from build123d import *

# Parameters (mm, degrees)
SKETCH1_R           = 1.755
SKETCH1_R_2         = 8
BOSS_EXTRUDE1_DEPTH = 3.175
SKETCH2_R           = 7.95936
SKETCH2_R_2         = 1.71436
BOSS_EXTRUDE2_DEPTH = 3.175


with BuildPart() as part:
    # Sketch1 → Boss-Extrude1 (new body)
    with BuildSketch(Plane.XY):
        Polygon((-50, 30), (-50, 33.175), (-70, 33.175), (-70, 30), (-90, 30), (-90, 33.175), (-110, 33.175), (-110, -33.175), (-90, -33.175), (-90, -30), (-70, -30), (-70, -33.175), (-50, -33.175), (-50, -30), (-30, -30), (-30, -33.175), (-10, -33.175), (-10, -30), (10, -30), (10, -33.175), (30, -33.175), (30, -30), (50, -30), (50, -33.175), (70, -33.175), (70, -30), (90, -30), (90, -33.175), (110, -33.175), (110, 33.175), (90, 33.175), (90, 30), (70, 30), (70, 33.175), (50, 33.175), (50, 30), (30, 30), (30, 33.175), (10, 33.175), (10, 30), (-10, 30), (-10, 33.175), (-30, 33.175), (-30, 30), align=None)
        with Locations((-65, -15)):
            Circle(SKETCH1_R, mode=Mode.SUBTRACT)
        with Locations((65, -15)):
            Circle(SKETCH1_R, mode=Mode.SUBTRACT)
        with Locations((-65, 15)):
            Circle(SKETCH1_R, mode=Mode.SUBTRACT)
        with Locations((-55, 0)):
            Circle(SKETCH1_R_2, mode=Mode.SUBTRACT)
        with BuildLine():
            ThreePointArc((2.5, -15), (0, -17.5), (-2.5, -15))
            Line((-2.5, -15), (-2.5, 15))
            ThreePointArc((-2.5, 15), (0, 17.5), (2.5, 15))
            Line((2.5, 15), (2.5, -15))
        make_face(mode=Mode.SUBTRACT)
        with Locations((55, 0)):
            Circle(SKETCH1_R_2, mode=Mode.SUBTRACT)
        with Locations((65, 15)):
            Circle(SKETCH1_R, mode=Mode.SUBTRACT)
    extrude(amount=BOSS_EXTRUDE1_DEPTH)

    # Sketch2 → Boss-Extrude2 (add)
    with BuildSketch(Plane.XY.offset(3.175)):
        Polygon((110.04064, -33.21564), (110.04064, 33.21564), (89.95936, 33.21564), (89.95936, 30.04064), (70.04064, 30.04064), (70.04064, 33.21564), (49.95936, 33.21564), (49.95936, 30.04064), (30.04064, 30.04064), (30.04064, 33.21564), (9.95936, 33.21564), (9.95936, 30.04064), (-9.95936, 30.04064), (-9.95936, 33.21564), (-30.04064, 33.21564), (-30.04064, 30.04064), (-49.95936, 30.04064), (-49.95936, 33.21564), (-70.04064, 33.21564), (-70.04064, 30.04064), (-89.95936, 30.04064), (-89.95936, 33.21564), (-110.04064, 33.21564), (-110.04064, -33.21564), (-89.95936, -33.21564), (-89.95936, -30.04064), (-70.04064, -30.04064), (-70.04064, -33.21564), (-49.95936, -33.21564), (-49.95936, -30.04064), (-30.04064, -30.04064), (-30.04064, -33.21564), (-9.95936, -33.21564), (-9.95936, -30.04064), (9.95936, -30.04064), (9.95936, -33.21564), (30.04064, -33.21564), (30.04064, -30.04064), (49.95936, -30.04064), (49.95936, -33.21564), (70.04064, -33.21564), (70.04064, -30.04064), (89.95936, -30.04064), (89.95936, -33.21564), align=None)
        with Locations((-55, 0)):
            Circle(SKETCH2_R, mode=Mode.SUBTRACT)
        with Locations((-65, 15)):
            Circle(SKETCH2_R_2, mode=Mode.SUBTRACT)
        with Locations((-65, -15)):
            Circle(SKETCH2_R_2, mode=Mode.SUBTRACT)
        with Locations((55, 0)):
            Circle(SKETCH2_R, mode=Mode.SUBTRACT)
        with Locations((65, 15)):
            Circle(SKETCH2_R_2, mode=Mode.SUBTRACT)
        with Locations((65, -15)):
            Circle(SKETCH2_R_2, mode=Mode.SUBTRACT)
        with BuildLine():
            Line((2.45936, -15), (2.45936, 15))
            ThreePointArc((2.45936, 15), (0, 17.45936), (-2.45936, 15))
            Line((-2.45936, 15), (-2.45936, -15))
            ThreePointArc((-2.45936, -15), (0, -17.45936), (2.45936, -15))
        make_face(mode=Mode.SUBTRACT)
    extrude(amount=-BOSS_EXTRUDE2_DEPTH)


solid = part.part
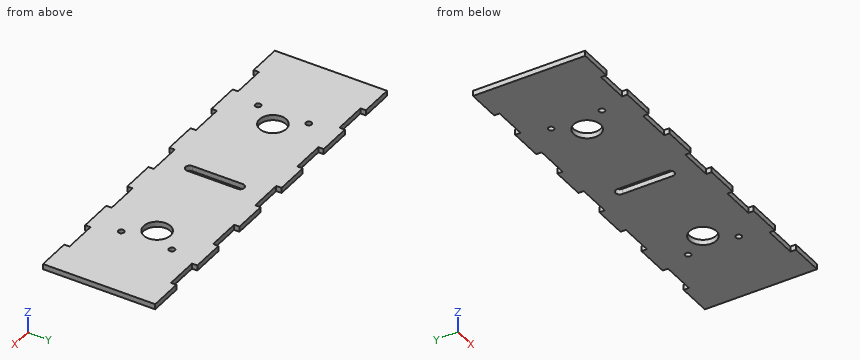
Could you check a few things on this model? Use its own coordinates, in mm. Round coordinates to 2 decimals unless told otherwise and drop trailing zeros. Order: outer loops, then holes, each group sorted by start corner. A loop starts at its lowest first (then second) coordinate and runs counter-clockwise, first axis right, second up.
(1) Imagine slicing it at B-B (y = 3). Write out the boundary of the cut face in (x, z) (3 decimals), plus the area to 3 significant figures.
Response values:
outline: (-110.041, 0) - (-62.372, 0) - (-62.372, 3.175) - (-110.041, 3.175) - close; (-47.628, 0) - (-2.459, 0) - (-2.459, 3.175) - (-47.628, 3.175) - close; (2.459, 0) - (47.628, 0) - (47.628, 3.175) - (2.459, 3.175) - close; (62.372, 0) - (110.041, 0) - (110.041, 3.175) - (62.372, 3.175) - close
area: 590 mm2
(2) Imagine slicing it at D-D (x = 0). Write out the boundary of the cut face in (y, z) (3 decimals), plus the area to 3 significant figures.
Response values:
outline: (-30.041, 0) - (-17.459, 0) - (-17.459, 3.175) - (-30.041, 3.175) - close; (17.459, 0) - (30.041, 0) - (30.041, 3.175) - (17.459, 3.175) - close
area: 79.9 mm2
(3) I'm going to push a flat-ended pin straight in: pin 1 (1 mm diameter, centred on x = -31.5, y = 18.5, fed in from -Z). Where does the tip first touch, or does it pass through?
Response values:
pin 1: stops at z = 0
(4) Imagine slicing it at A-A (x = -55). Write out the boundary of the cut face in (y, z) (3 decimals), plus the area to 3 significant figures.
Response values:
outline: (-33.216, 0) - (-7.959, 0) - (-7.959, 3.175) - (-33.216, 3.175) - close; (7.959, 0) - (33.216, 0) - (33.216, 3.175) - (7.959, 3.175) - close
area: 160 mm2
(5) Please list where these lines run through material, in increasing order: line 1 along Y through (x, z) = (-65, 1.6); line 2 along X through (y, z) = (-10, 2.4); line 3 along Y through (x, z) = (-55, 1.25).
Response values:
line 1: y = -33.22 to -16.71, -13.29 to 13.29, 16.71 to 33.22
line 2: x = -110.04 to -2.46, 2.46 to 110.04
line 3: y = -33.22 to -7.96, 7.96 to 33.22
(6) Imagine slicing it at C-C (z = 1). Count the separate pieces of the cut face and the enclosed holes in it, plus the area to 3 significant figures.
Response values:
separate pieces: 1
enclosed holes: 7
area: 13,400 mm2
